from build123d import *

# Parameters (mm, degrees)
SKETCH1_R           = 3
BOSS_EXTRUDE1_DEPTH = 43.942


with BuildPart() as part:
    # Sketch1 → Boss-Extrude1 (new body)
    with BuildSketch(Plane(origin=(0, 0, 0), x_dir=(1, 0, 0), z_dir=(0, 1, 0))):
        with BuildLine():
            ThreePointArc((-11.995636707, -5.54), (-9.328503626, -2.300965424), (-5.819871132, 0))
            ThreePointArc((-5.819871132, 0), (0, 1.27), (5.819871133, 0))
            ThreePointArc((5.819871133, 0), (9.328503626, -2.300965424), (11.995636707, -5.54))
            Line((11.995636707, -5.54), (12.7, -5.54))
            ThreePointArc((12.7, -5.54), (18.24, 0), (12.7, 5.54))
            Line((12.7, 5.54), (-12.7, 5.54))
            ThreePointArc((-12.7, 5.54), (-18.24, 0), (-12.7, -5.54))
            Line((-12.7, -5.54), (-11.995636707, -5.54))
        make_face()
        with Locations(Location((-12.7, 0, 0), (0, 0, 90))):
            Circle(SKETCH1_R, mode=Mode.SUBTRACT)
        with BuildLine():
            ThreePointArc((15.7, 0), (12.7, -3), (9.7, 0))
            ThreePointArc((9.7, 0), (12.7, 3), (15.7, 0))
        make_face(mode=Mode.SUBTRACT)
    extrude(amount=BOSS_EXTRUDE1_DEPTH)


solid = part.part
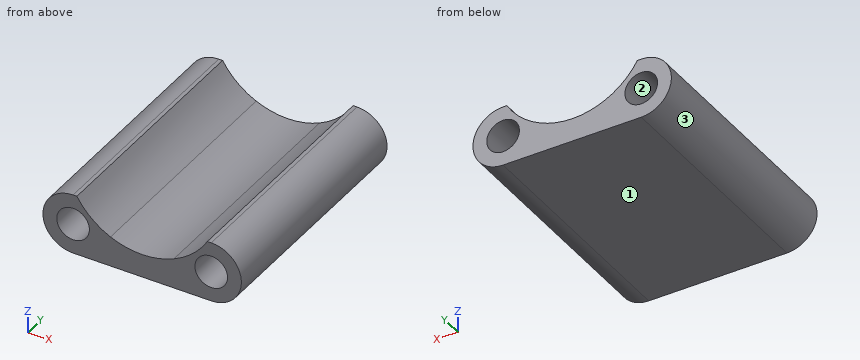
Can you work these out from the model? Positions are in its coordinate system, mm. Face numbers are marked on the shaded views. Coordinates: 2 decimals unless noted, no trailing zeros. Write each loop counter-clockwise with the first axis right and the second up, starting at its lowest first coordinate (ties: lowest second). Pieces come first, ordered by that corner, then holes. Notation, with made-up numbers: (51, 79) - (105, 79) arc R21 ccw to (105, 101) - close; hole circle Ø9 at (6.25, -20). An arc over 180 degrees is marked (long way). Return JSON: item names as keys, results as strings. Group by question number.
Item 1: If we section it at D-D (x = -7): Write out the boundary of the cut face in (y, z), then the cut area to 3 significant figures.
Item 2: I'm going to push flat-ended pins straight in: pin 1 Ø3.5 at (x, z) = (12.7, 0) entering from +Y; pin 2 Ø5 at (x, z) = (7.5, 0) entering from -Y; pin 3 Ø2 at (y, z) = (10.5, 3) entering from -X; pin 4 Ø2 at (y, z) = (38.5, -1.5) entering from -X. Where does each tip first touch, or does it pass through?
Item 3: Please list where these lines run through material, in increasing order: probe 1 along X at (y, z) = (7, 2.75); probe 2 along Z at (x, y) = (-12.7, 23); probe 3 along X at (y, z) = (34.5, 0.25).
Item 4: We'd pull the mould along X, two halves only. Please class the marked faces 1, 2 and 3: pulls with the +X half, pulls with the -X half, needs draft (parallel to the pull), parting line crosses it, or undercut.
Item 5: If we section it at B-B (z = -2.5): Write out the boundary of the cut face in (x, y).
Item 6: If we section it at A-A (y = 8): Write out the boundary of the cut face in (x, z), then the cut area to 3 significant figures.
Item 7: If we section it at C-C (z = 4): Write out the boundary of the cut face in (x, y).
Return value:
{
 "1": {"outline": "(0, -5.54) - (43.94, -5.54) - (43.94, 0.61) - (0, 0.61) - close", "area": "270 mm^2"},
 "2": {"pin 1": "passes through", "pin 2": "stops at y = 0", "pin 3": "stops at x = -17.87", "pin 4": "stops at x = -18.22"},
 "3": {"probe 1": "x = -17.51 to -13.9, -11.5 to -9.81, 9.81 to 11.5, 13.9 to 17.51", "probe 2": "z = -5.54 to -3, 3 to 5.54", "probe 3": "x = -18.23 to -15.69, -9.71 to -6.34, 6.34 to 9.71, 15.69 to 18.23"},
 "4": {"face 1": "needs draft", "face 2": "undercut", "face 3": "pulls with the -X half"},
 "5": {"outline": "(-17.64, 0) - (-14.36, 0) - (-14.36, 43.94) - (-17.64, 43.94) - close; (-11.04, 0) - (11.04, 0) - (11.04, 43.94) - (-11.04, 43.94) - close; (14.36, 0) - (17.64, 0) - (17.64, 43.94) - (14.36, 43.94) - close"},
 "6": {"outline": "(-12.7, -5.54) - (12.7, -5.54) arc R5.54 ccw to (12.7, 5.54) - (12, 5.54) arc R13.97 cw to (-12, 5.54) - (-12.7, 5.54) arc R5.54 ccw to start; hole circle Ø6 at (-12.7, 0); hole circle Ø6 at (12.7, 0)", "area": "206 mm^2"},
 "7": {"outline": "(-16.53, 0) - (-10.93, 0) - (-10.93, 43.94) - (-16.53, 43.94) - close; (10.93, 0) - (16.53, 0) - (16.53, 43.94) - (10.93, 43.94) - close"}
}
